from build123d import *

# Parameters (mm, degrees)
DIAM_TRE_DU_PER_AGE_9_0_9_1_D     = 9
DIAM_TRE_DU_PER_AGE_9_0_9_1_DEPTH = 3
D_GAGEMENT_M31_D                  = 3.332
D_GAGEMENT_M31_DEPTH              = 16
D_GAGEMENT_M31_TIP                = 1.001033791
D_GAGEMENT_M1001_D                = 110
D_GAGEMENT_M1001_DEPTH            = 35
CHANFREIN1_SIZE                   = 0.2
CHANFREIN2_SIZE                   = 1


with BuildPart() as part:
    # Esquisse1 → Révolution1 (revolve)
    with BuildSketch(Plane(origin=(0, 0, 0), x_dir=(1, 0, 0), z_dir=(0, 1, 0))):
        Polygon((87.5, 159.225), (0, 159.225), (0, 114.225), (75.15, 114.225), (75.15, 121.425), (70.15, 121.425), (70.15, 131.025), (75.15, 131.025), (75.15, 137.425), (70.15, 137.425), (70.15, 147.025), (75.15, 147.025), (75.15, 149.225), (87.5, 149.225), align=None)
    revolve(axis=Axis((0, 0, -159.225), (0, 0, 1)))

    # Diamètre du perçage Ø9.0 (9)1
    with Locations(Plane.XY.offset(-149.225)):
        with Locations((-87.5, 0), (0, 87.5), (0, -87.5), (87.5, 0)):
            Hole(DIAM_TRE_DU_PER_AGE_9_0_9_1_D / 2, depth=DIAM_TRE_DU_PER_AGE_9_0_9_1_DEPTH)

    # Dégagement M31
    with Locations(Plane.XY.offset(-114.225)):
        with Locations((-65, 0), (65, 0), (0, 65), (0, -65)):
            Hole(D_GAGEMENT_M31_D / 2, depth=D_GAGEMENT_M31_DEPTH)
            with Locations((0, 0, -(D_GAGEMENT_M31_DEPTH + D_GAGEMENT_M31_TIP / 2))):  # 118° drill point
                Cone(0, D_GAGEMENT_M31_D / 2, D_GAGEMENT_M31_TIP, mode=Mode.SUBTRACT)

    # Dégagement M1001
    with Locations(Plane.XY.offset(-114.225)):
        with Locations((0, 0)):
            Hole(D_GAGEMENT_M1001_D / 2, depth=D_GAGEMENT_M1001_DEPTH)

    # Chanfrein1
    chanfrein1_edges = [part.edges().sort_by_distance(p)[0] for p in [
        (-75.15, 0, -147.025),
        (-75.15, 0, -137.425),
        (-75.15, 0, -131.025),
        (-75.15, 0, -121.425),
    ]]
    chamfer(chanfrein1_edges, length=CHANFREIN1_SIZE)

    # Chanfrein2
    chanfrein2_edges = [part.edges().sort_by_distance(p)[0] for p in [
        (-75.15, 0, -114.225),
        (-87.5, 0, -159.225),
    ]]
    chamfer(chanfrein2_edges, length=CHANFREIN2_SIZE)


solid = part.part
Geometry: final body of the model. Coordinates: model frame, mm. A direction names the side the tool comes from. Give positions to 0.01 mm unless a question says otherwise; leave off trailing zeros. Loops run counter-clockwise (first coordinate to the right, second up) from the corner with the lowest first, then second, coordinate; pieces in that order, holes last. Notation, with made-up numbers: M 38.5,84.25 L 70.5,84.25 A21 cw 70.5,90.25 Z; hole C 76,72.5 d7. An arc over 180 degrees is marked long. Put each result on its own line as item: value. Start each with the question number.
1) Cut plane B-B (z = -144). Output: boundary loops of the cut face in (x, y).
2) Ray query, line 1 along Y through (x, z) = (0, -122.25); line 2 along Z through (x, y) = (-62, -37) (3 decimals); line 3 along Z through (x, y) = (3.5, -76) (3 decimals). Return the intervals inside material, ascending.
3) Contact query for flat-ended pins moving along their axis: pin 1 (5 mm diameter, centred on x = 85, y = 0, fed in from +Z) (3 decimals); pin 2 (6 mm diameter, centred on y = 52.5, z = -141.5, fed in from -X); pin 3 (4 mm diameter, centred on y = -23.5, z = -138, fed in from +X); pin 4 (4.5 mm diameter, centred on x = -65, y = 0, fed in from +Z) (3 decimals). Output: stop coordinate, or through.
4) Pull-direction query (Y, two-part tool) for faces 1 (the flat face through (-50, -50, -131.025)), 2 (the cylindrical face through (83.46, 26.28, -153.79)), 3 (the cylindrical face through (11.923, -53.692, -131.97)); classes: pulls with the +Y half, pulls with the -Y half, needs draft (parallel to the pull), parting line crosses it, or undercut.
5) Cut plane A-A (z = -128). Output: boundary loops of the cut face in (x, y).
6) Access query for faces 4 (the flat face through (0, -86, -152.225)), 5 (the flat face through (86, 0, -152.225)), 6 (the flat face through (50, -50, -121.425)), 7 (the cylindrical face through (69.42, -28.78, -118.27)). Directions: +Z, -Z, +X, -X, +Y, -Y. A direction counts if a zero-diameter tool reaches every point of the face in a straight line with its end or side. Return the directions, or none.
Verdict:
1. outline: C 0,0 d140.3; hole C 0,0 d110
2. line 1: -70.15 to -66.67, -63.33 to -55, 55 to 63.33, 66.67 to 70.15
2. line 2: -159.225 to -147.025, -137.425 to -131.025, -121.425 to -114.225
2. line 3: -159.225 to -149.225
3. pin 1: z = -149.225
3. pin 2: x = -49.71
3. pin 3: x = 71.96
3. pin 4: z = -114.225
4. face 1: needs draft
4. face 2: parting line crosses it
4. face 3: undercut
5. outline: C 0,0 d140.3; hole C -65,0 d3.33; hole C 0,0 d110; hole C 0,-65 d3.33; hole C 0,65 d3.33; hole C 65,0 d3.33
6. face 4: +Z, -Y
6. face 5: +Z, +X
6. face 6: none
6. face 7: +Z
